```python
from build123d import *

# Parameters (mm, degrees)
CROQUIS1_R              = 15.5
CROQUIS1_R_2            = 10
SALIENTE_EXTRUIR1_DEPTH = 21
CROQUIS2_R              = 23
SALIENTE_EXTRUIR2_DEPTH = 5
CROQUIS3_R              = 5
CORTAR_EXTRUIR1_DEPTH   = 5
CORTAR_EXTRUIR2_START   = -5
CROQUIS4_R              = 23
CROQUIS4_R_2            = 20
CORTAR_EXTRUIR2_DEPTH   = 5


with BuildPart() as part:
    # Croquis1 → Saliente-Extruir1 (new body)
    with BuildSketch(Plane(origin=(0, 0, 0), x_dir=(1, 0, 0), z_dir=(0, 1, 0))):
        with Locations(Location((0, 0, 0), (0, 0, 90))):
            Circle(CROQUIS1_R)
        with Locations(Location((0, 0, 0), (0, 0, 90))):
            Circle(CROQUIS1_R_2, mode=Mode.SUBTRACT)
    extrude(amount=SALIENTE_EXTRUIR1_DEPTH)

    # Croquis2 → Saliente-Extruir2 (add)
    with BuildSketch(Plane(origin=(0, 21, 0), x_dir=(1, 0, 0), z_dir=(0, 1, 0))):
        with Locations(Location((0, 0, 0), (0, 0, 270))):
            Circle(CROQUIS2_R)
    extrude(amount=SALIENTE_EXTRUIR2_DEPTH)

    # Croquis3 → Cortar-Extruir1 (cut)
    with BuildSketch(Plane(origin=(0, 26, 0), x_dir=(1, 0, 0), z_dir=(0, 1, 0))):
        with Locations((0, 23)):
            Circle(CROQUIS3_R)
        with Locations((13.519060803, 18.607390871)):
            Circle(CROQUIS3_R)
        with Locations((21.874299875, 7.107390871)):
            Circle(CROQUIS3_R)
        with Locations((21.874299875, -7.107390871)):
            Circle(CROQUIS3_R)
        with Locations((13.519060803, -18.607390871)):
            Circle(CROQUIS3_R)
        with Locations((0, -23)):
            Circle(CROQUIS3_R)
        with Locations((-13.519060803, -18.607390871)):
            Circle(CROQUIS3_R)
        with Locations((-21.874299875, -7.107390871)):
            Circle(CROQUIS3_R)
        with Locations((-21.874299875, 7.107390871)):
            Circle(CROQUIS3_R)
        with Locations((-13.519060803, 18.607390871)):
            Circle(CROQUIS3_R)
    extrude(amount=-CORTAR_EXTRUIR1_DEPTH, mode=Mode.SUBTRACT)

    # Croquis4 → Cortar-Extruir2 (cut)
    with BuildSketch(Plane(origin=(0, 26, 0), x_dir=(1, 0, 0), z_dir=(0, 1, 0)).offset(CORTAR_EXTRUIR2_START)):
        Circle(CROQUIS4_R)
        Circle(CROQUIS4_R_2, mode=Mode.SUBTRACT)
    extrude(amount=CORTAR_EXTRUIR2_DEPTH, mode=Mode.SUBTRACT)


solid = part.part
```
The model under review builds one solid part; all positions refer to its coordinate system, in mm. A direction names the side the tool comes from. Round coordinates to 2 decimals unless told otherwise and drop trailing zeros. Order: outer loops, then holes, each group sorted by start corner. A loop starts at its lowest first (then second) coordinate and runs counter-clockwise, first axis right, second up.
Item 1: To check wall thickness, follow probe 1 along X at (y, z) = (15.5, 0); probe 2 along Y at (x, z) = (-6, -4.5); probe 3 along X at (y, z) = (13, 1). State the ranges of each line that lie inside material, in increasing order.
Working result:
probe 1: x = -15.5 to -10, 10 to 15.5
probe 2: y = 21 to 26
probe 3: x = -15.47 to -9.95, 9.95 to 15.47
Item 2: Add section D-D, the plane z = -12.5. State the section outline as (x, y) points, and give its area (3 significant figures).
Working result:
outline: (-15.61, 21) - (-9.17, 21) - (-9.17, 0) - (9.17, 0) - (9.17, 21) - (15.61, 21) - (15.61, 26) - (-15.61, 26) - close
area: 541 mm2
Item 3: Add section A-A, the plane x = 0. State the section outline as (y, z) points, and give its area (3 significant figures).
Working result:
outline: (0, -15.5) - (21, -15.5) - (21, -18) - (26, -18) - (26, 18) - (21, 18) - (21, 15.5) - (0, 15.5) - (0, 10) - (21, 10) - (21, -10) - (0, -10) - close
area: 411 mm2
Item 4: For pin 1 (3 mm diameter, centred on x = 9.5, y = 7.5, fed in from -Z); pin 2 (10 mm diameter, centred on x = 1, z = 4.5, fed in from -Y); pin 3 (10 mm diameter, centred on y = 13, z = -10.5, fed in from -X), all flat-tipped, find the tip position at first contact; note any pin that passes through.
Working result:
pin 1: stops at z = -13.28
pin 2: stops at y = 21
pin 3: stops at x = -14.49
Item 5: Add section C-C, the plane y = 7. State the section outline as (x, z) points.
Working result:
outline: circle Ø31 at (0, 0); hole circle Ø20 at (0, 0)
Item 6: Machinability: for faces 1 (the flat face through (0, 21, 0)), 2 (the cylindrical face through (16, 23, -12)), which of the approach directions +Z, -Z, +X, -X, +Y, -Y give a long, thin tool a straight path to every point of the face, cutting with its end or side? Answer none if there is none.
Working result:
face 1: -Y
face 2: -Z, +X, +Y, -Y
Item 7: Add section B-B, the plane z = 0. State the section outline as (x, y) points, and give its area (3 significant figures).
Working result:
outline: (-20, 21) - (-15.5, 21) - (-15.5, 0) - (-10, 0) - (-10, 21) - (10, 21) - (10, 0) - (15.5, 0) - (15.5, 21) - (20, 21) - (20, 26) - (-20, 26) - close
area: 431 mm2
Item 8: Draft analysis for pull direction Z (two halves, no side actions). For faces 3 (the cylindrical face through (17, 24, 6)), 4 (the flat face through (0, 26, 0)), 5 (the cylindrical face through (-16, 23, 12)), state which applies: released by +Z, released by -Z, zero draft, split by the parting line, or undercut.
Working result:
face 3: undercut
face 4: zero draft
face 5: released by +Z
